Can you work these out from the model? Positions are in its coordinate system, mm. Round coordinates to 2 decimals unless told otherwise and drop trailing zeros. Loops run counter-clockwise (first coordinate to the right, second up) from the corner with the lowest first, then second, coordinate; pieces in that order, holes last. Notation, with made-up numbers: (-29.75, 85) -> (-0.75, 85) arc R16 ccw to (-0.75, 114) -> close; hole circle Ø2 at (22.25, 53.5). An arc over 180 degrees is marked (long way). Use a Markdown table: item, result.
from build123d import *

# Parameters (mm, degrees)
SZKIC1_R                    = 40
SZKIC1_R_2                  = 30
DODANIE_WYCI_GNI_CIE1_DEPTH = 70
SZKIC2_R                    = 130
SZKIC2_R_2                  = 120
DODANIE_WYCI_GNI_CIE2_DEPTH = 70
DODANIE_WYCI_GNI_CIE3_START = -70
DODANIE_WYCI_GNI_CIE3_DEPTH = 70
SZYK_KO_OWY1_COUNT          = 16
SZKIC4_R                    = 130
SZKIC4_R_2                  = 120
WYTNIJ_WYCI_GNI_CIE1_DEPTH  = 70


with BuildPart() as part:
    # Szkic1 → Dodanie-wyci_gni_cie1 (new body)
    with BuildSketch(Plane.XY):
        with Locations((-26.191385705, 0)):
            Circle(SZKIC1_R)
        with Locations((-26.191385705, 0)):
            Circle(SZKIC1_R_2, mode=Mode.SUBTRACT)
    extrude(amount=DODANIE_WYCI_GNI_CIE1_DEPTH)



with BuildPart() as body_2:
    # Szkic2 → Dodanie-wyci_gni_cie2 (new body)
    with BuildSketch(Plane.XY.offset(70)):
        with Locations((-26.191385705, 0)):
            Circle(SZKIC2_R)
        with Locations((-26.191385705, 0)):
            Circle(SZKIC2_R_2, mode=Mode.SUBTRACT)
    extrude(amount=-DODANIE_WYCI_GNI_CIE2_DEPTH)


with BuildPart() as part_1:
    add(part.part)

    add(body_2.part)  # Dodanie-wyci_gni_cie3 merges body 2
    # Szkic3 → Dodanie-wyci_gni_cie3 (add)
    with BuildSketch(Plane.XY.offset(70).offset(DODANIE_WYCI_GNI_CIE3_START)):
        with BuildLine():
            ThreePointArc((-66.191385705, 0), (-106.191385705, 14.477555095), (-146.191385705, 0))
            ThreePointArc((-146.191385705, 0), (-146.165341212, -2.5), (-146.087219038, -4.998914813))
            ThreePointArc((-146.087219038, -4.998914813), (-105.468199385, 8.892478563), (-65.578885705, -6.973151637))
            ThreePointArc((-65.578885705, -6.973151637), (-66.037966486, -3.5), (-66.191385705, 0))
        make_face()
    dodanie_wyci_gni_cie3 = extrude(amount=DODANIE_WYCI_GNI_CIE3_DEPTH)

    # Szyk ko_owy1: Dodanie-wyci_gni_cie3 ×16 about axis
    szyk_ko_owy1_axis = Axis((-26.191385705, 0, 0), (0, 0, 1))
    for i in range(1, SZYK_KO_OWY1_COUNT):
        add(dodanie_wyci_gni_cie3.rotate(szyk_ko_owy1_axis, i * 360 / SZYK_KO_OWY1_COUNT))

    # Szkic4 → Wytnij-wyci_gni_cie1 (cut)
    with BuildSketch(Plane.XY.offset(70)):
        with Locations((-26.191385705, 0)):
            Circle(SZKIC4_R)
        with Locations((-26.191385705, 0)):
            Circle(SZKIC4_R_2, mode=Mode.SUBTRACT)
    extrude(amount=-WYTNIJ_WYCI_GNI_CIE1_DEPTH, mode=Mode.SUBTRACT)


solid = part_1.part
1. I want a section at C-C (y = -58). Please give me the cut outline in (x, z).
Answer sheet:
| item | result |
|---|---|
| outline | (-102.17, 0) -> (-95.77, 0) -> (-95.77, 70) -> (-102.17, 70) -> close; (-64.69, 0) -> (-57.84, 0) -> (-57.84, 70) -> (-64.69, 70) -> close; (-36.67, 0) -> (-30.75, 0) -> (-30.75, 70) -> (-36.67, 70) -> close; (-13.66, 0) -> (-8.11, 0) -> (-8.11, 70) -> (-13.66, 70) -> close; (12.82, 0) -> (19.81, 0) -> (19.81, 70) -> (12.82, 70) -> close |
2. If we mould it in two halves opening along X, with no side actions, what happens to faces 1 (the flat face through (-53, -17, 0)), 2 (the cylindrical face through (-43.2, 78.89, 34.51))? For each: +X half, -X half, draft (parallel to the pull), parting line (faces both ways), or undercut.
Answer sheet:
| item | result |
|---|---|
| face 1 | draft |
| face 2 | undercut |
3. I want a section at D-D (x = -95.5). Please give me the cut outline in (y, z).
Answer sheet:
| item | result |
|---|---|
| outline | (-57.63, 0) -> (-48.98, 0) -> (-48.98, 70) -> (-57.63, 70) -> close; (-19.8, 0) -> (-14.02, 0) -> (-14.02, 70) -> (-19.8, 70) -> close; (7.84, 0) -> (13.56, 0) -> (13.56, 70) -> (7.84, 70) -> close; (38.32, 0) -> (44.37, 0) -> (44.37, 70) -> (38.32, 70) -> close; (76.16, 0) -> (81.4, 0) -> (81.4, 70) -> (76.16, 70) -> close |
4. Will these pins go through, and if not, where does the flat tip stop? pin 1 Ø6 at (y, z) = (-39.5, 8) entering from -X; pin 2 Ø2 at (y, z) = (-83, 29) entering from -X; pin 3 Ø3 at (x, y) = (31, 41.5) entering from -Z; pin 4 Ø2 at (y, z) = (90, 15.5) entering from +X.
Answer sheet:
| item | result |
|---|---|
| pin 1 | stops at x = -135.12 |
| pin 2 | stops at x = -110.96 |
| pin 3 | stops at z = 0 |
| pin 4 | stops at x = 22.54 |
5. I want a section at B-B (y = 105). Please give me the cut outline in (x, z), plus the area to 3 significant figures.
Answer sheet:
| item | result |
|---|---|
| outline | (-70.46, 0) -> (-62.97, 0) -> (-62.97, 70) -> (-70.46, 70) -> close; (-22.21, 0) -> (-16.93, 0) -> (-16.93, 70) -> (-22.21, 70) -> close; (16.85, 0) -> (21.25, 0) -> (21.25, 70) -> (16.85, 70) -> close |
| area | 1,200 mm² |
6. I want a section at A-A (x = -122). Please give me the cut outline in (y, z), plus the area to 3 significant figures.
Answer sheet:
| item | result |
|---|---|
| outline | (-33.89, 0) -> (-27.19, 0) -> (-27.19, 70) -> (-33.89, 70) -> close; (7.06, 0) -> (12.45, 0) -> (12.45, 70) -> (7.06, 70) -> close; (43.86, 0) -> (48.65, 0) -> (48.65, 70) -> (43.86, 70) -> close |
| area | 1,180 mm² |
7. I need wall thicknesses on line 1 (Y direction, x = -75, z = 17.5); line 2 (Y direction, x = -112.5, z = 54); line 3 (Y direction, x = -135.5, z = 64). Which ranges of each line are inside material? Lowest first, please.
Answer sheet:
| item | result |
|---|---|
| line 1 | y = -39.99 to -33.78, -18.22 to -12.84, 0.01 to 6.14, 23.26 to 31.15, 61.31 to 69.15, 107.91 to 109.63 |
| line 2 | y = -26.85 to -20.58, 8.67 to 14.16, 43.26 to 48.46, 81.01 to 83.37 |
| line 3 | y = -49.51 to -43.13, 1.95 to 7.18, 42.17 to 46.38 |
